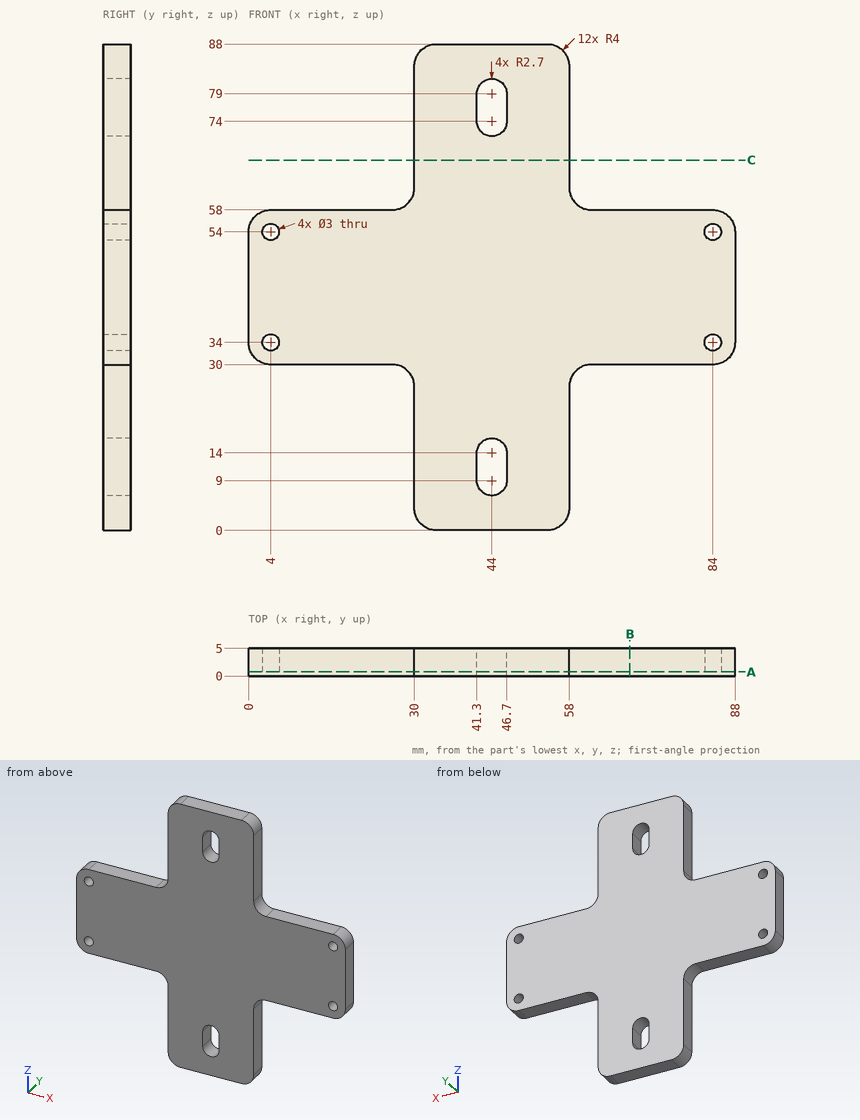
Job drawing, mm, ordinate dimensions from the low corner. One solid piece. Round coordinates to 2 decimals unless told otherwise and drop trailing zeros. Write each loop counter-clockwise with the first axis right and the second up, starting at its lowest first coordinate (ties: lowest second). Pieces come first, ordered by that corner, then holes. Notation, with made-up numbers: M 57,76 L 92,76 A17 ccw 92,92 Z; hole C 18,-1 d9. An arc over 180 degrees is marked long. Return JSON: item names as keys, results as strings. Group by question number.
(1) Saw through at B-B on x = 69. Write the cut outline in (y, z), then the cut area to 3 significant figures.
(2) Drill centre lines: probe 1 along Z at (x, y) = (4, 1.7); probe 2 along X at (y, z) = (1.3, 54); probe 3 along X at (y, z) = (4.7, 53.5). Where is each one in solid material? Low to high.
(3) Saw through at A-A on y = 0.75. Count the separate pieces of the cut face and the enclosed holes in it, then the cut area to 3 significant figures.
(4) Pin check, flat tips, straight feed: pin 1 Ø1.5 at (y, z) = (3.5, 10.5) entering from +X; pin 2 Ø1.5 at (y, z) = (2, 70) entering from -X; pin 3 Ø3 at (x, y) = (31, 2) entering from -Z. Stop position of each tip, or through.
(5) Saw through at C-C on z = 67. Write the cut outline in (x, y), then the cut area to 3 significant figures.
Returned:
{
 "1": {"outline": "M 0,30 L 5,30 L 5,58 L 0,58 Z", "area": "140 mm²"},
 "2": {"probe 1": "30 to 32.5, 35.5 to 52.5, 55.5 to 58", "probe 2": "0 to 2.5, 5.5 to 82.5, 85.5 to 88", "probe 3": "0 to 2.59, 5.41 to 82.59, 85.41 to 88"},
 "3": {"separate pieces": "1", "enclosed holes": "6", "area": "4,000 mm²"},
 "4": {"pin 1": "x = 58", "pin 2": "x = 30", "pin 3": "z = 0.29"},
 "5": {"outline": "M 30,0 L 58,0 L 58,5 L 30,5 Z", "area": "140 mm²"}
}
